For this review, take the finished solid that the model builds, in its own axes (mm). Round coordinates to 2 decimals unless told otherwise and drop trailing zeros. Loops run counter-clockwise (first coordinate to the right, second up) from the corner with the lowest first, then second, coordinate; pieces in that order, holes last.
1. To check wall thickness, follow line 1 along Y through (x, z) = (-384, 0.9); line 2 along X through (y, z) = (8.5, 2.05); line 3 along X through (y, z) = (20, 1.1). State the ranges of each line that lie inside material, in increasing order.
2. Consider section B-B on z = 2.3. State how many separate pieces and enclosed holes the cut face has, then the cut area to 3 significant figures.
3. Consider section A-A on x = -354. State the section outline as (y, z) points, then the cut area to 3 significant figures.
4. Clearance check with flat-ended pins moving along their axes: pin 1 Ø20.5 at (x, y) = (-324, 67) entering from -Z; pin 2 Ø3 at (x, y) = (-224.5, 9) entering from -Z. State where each tip first meets the part, or that it passes through.
from build123d import *

# Parameters (mm, degrees)
SCHIZZO1_W                   = 449
SCHIZZO1_H                   = 94
SCHIZZO1_R                   = 7.8
SCHIZZO1_R_2                 = 2
SCHIZZO1_R_3                 = 6
ESTRUSIONE_ESTRUSIONE1_DEPTH = 4


with BuildPart() as part:
    # Schizzo1 → Estrusione-Estrusione1 (new body)
    with BuildSketch(Plane.XY):
        with Locations((-224.5, 47)):
            Rectangle(SCHIZZO1_W, SCHIZZO1_H)
        with Locations(Location((-384, 27, 0), (0, 0, 180))):
            Circle(SCHIZZO1_R, mode=Mode.SUBTRACT)
        with Locations((-9, 47)):
            Circle(SCHIZZO1_R_2, mode=Mode.SUBTRACT)
        with Locations((-224.5, 85)):
            Circle(SCHIZZO1_R_2, mode=Mode.SUBTRACT)
        with Locations(Location((-440, 47, 0), (0, 0, 180))):
            Circle(SCHIZZO1_R_2, mode=Mode.SUBTRACT)
        with Locations(Location((-224.5, 9, 0), (0, 0, 180))):
            Circle(SCHIZZO1_R_2, mode=Mode.SUBTRACT)
        with Locations((-324, 27)):
            Circle(SCHIZZO1_R, mode=Mode.SUBTRACT)
        with Locations(Location((-324, 67, 0), (0, 0, 180))):
            Circle(SCHIZZO1_R, mode=Mode.SUBTRACT)
        with Locations((-336.75, 85)):
            Circle(SCHIZZO1_R_2, mode=Mode.SUBTRACT)
        with Locations((-384, 67)):
            Circle(SCHIZZO1_R, mode=Mode.SUBTRACT)
        with Locations(Location((-336.75, 9, 0), (0, 0, 180))):
            Circle(SCHIZZO1_R_2, mode=Mode.SUBTRACT)
        with Locations((-112.25, 9)):
            Circle(SCHIZZO1_R_2, mode=Mode.SUBTRACT)
        with Locations(Location((-112.25, 85, 0), (0, 0, 180))):
            Circle(SCHIZZO1_R_2, mode=Mode.SUBTRACT)
        with Locations((-354, 47)):
            Circle(SCHIZZO1_R_3, mode=Mode.SUBTRACT)
    extrude(amount=ESTRUSIONE_ESTRUSIONE1_DEPTH)


solid = part.part
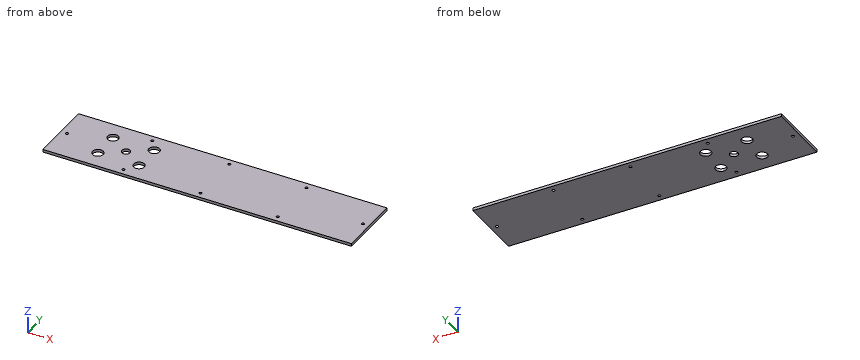
Resolved:
1. line 1: y = 0 to 19.2, 34.8 to 59.2, 74.8 to 94
1. line 2: x = -449 to -338.69, -334.81 to -226.44, -222.56 to -114.19, -110.31 to 0
1. line 3: x = -449 to -387.44, -380.56 to -327.44, -320.56 to 0
2. separate pieces: 1
2. enclosed holes: 13
2. area: 41,200 mm2
3. outline: (0, 0) - (41, 0) - (41, 4) - (0, 4) - close; (53, 0) - (94, 0) - (94, 4) - (53, 4) - close
3. area: 328 mm2
4. pin 1: stops at z = 0
4. pin 2: passes through
